Source: CAD feature listing. Evaluate the final solid. Frame: model axes, mm. Face numbers are marked on the shaded views. A direction names the side the tool comes from. Round coordinates to 2 decimals unless told otherwise and drop trailing zeros. Write each loop counter-clockwise with the first axis right and the second up, starting at its lowest first coordinate (ties: lowest second). Pieces come first, ordered by that corner, then holes.
Autodesk Inventor part; units mm, degrees
ref_plane "YZ Plane" through (0, 0, 0) normal (1, 0, 0) x (0, 1, 0)
ref_plane "XZ Plane" through (0, 0, 0) normal (0, 1, 0) x (-1, 0, 0)
ref_plane "XY Plane" through (0, 0, 0) normal (0, 0, 1) x (1, 0, 0)
sketch "Sketch1" plane through (0, 0, 0) normal (0, 1, 0) x (-1, 0, 0)
  circle A0 centre (0, 0) radius 15
  circle A1 centre (0, 0) radius 23.5
  circle A2 centre (0, 0) radius 15.5
  circle A3 centre (0, 0) radius 23
  dimension "d0" = 30
  dimension "d1" = 47
  dimension "d2" = 0.5
  dimension "d3" = 0.5
extrude "Extrusion1" add sketch "Sketch1" along normal mid plane 11 contours A1 | A2 | A3
extrude "Extrusion2" cut sketch "Sketch1" along normal mid plane 4
properties part number "Thrust Bearing 51106 - 30x47x11mm" material "Stainless Steel"
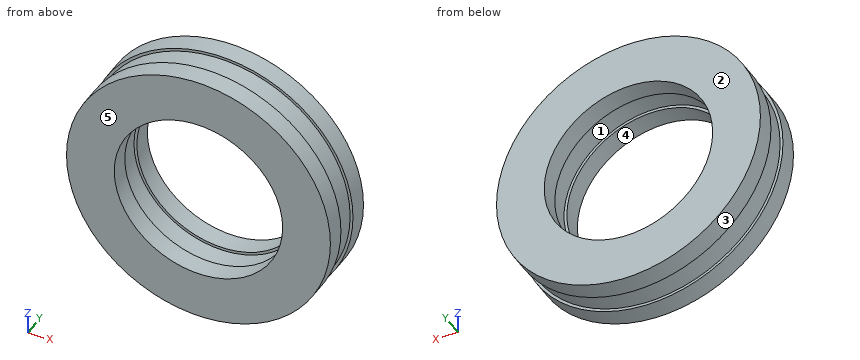
Q1. Section query D-D, the plane x = 21.5. Output: boundary loops of the cut face in (y, z).
Q2. Line query: line 1 (Z direction, x = 0, y = 4.05); line 2 (X direction, y = -4.25, z = -12.5); line 3 (Z direction, x = -5, y = -3.75). Output: solid intervals per line, ascending.
Q3. Set-up query: the marked faces 1 and 2. Return all of +Z, -Z, +X, -X, +Y, -Y with unobstructed straight access to the full face (end or side cutting, diameter ignored); none if empty.
Q4. Section query B-B, the plane x = 0. Output: boundary loops of the cut face in (y, z).
Q5. Mould query, pull axis Z, two halves, no side actions, for the marked faces 3, 4 and 5. Classes: pulls with the +Z half, pulls with the -Z half, needs draft (parallel to the pull), parting line crosses it, or undercut.
Q6. Pin query (flat end, axial travel): P1, Ø4, axis at x = -13.5, y = -2.5, coming from the -Z side; P2, Ø2, axis at x = 0.5, y = -0.5, coming from the +Z side; P3, Ø25, axis at x = -5.5, z = 4, coming from the +Y side; P4, Ø1, axis at y = 4, z = -17.5, coming from the +X side (3 decimals). Return the tip coordinate at first contact, or that it passes through.
Q7. Section query A-A, the plane z = 0. Output: boundary loops of the cut face in (x, y).
Q8. Section query C-C, the plane y = 4.25. Output: boundary loops of the cut face in (x, z), and give its area (3 significant figures).
Filled in:
1. outline: (-5.5, -9.49) - (-2, -9.49) - (-2, -8.17) - (2, -8.17) - (2, -9.49) - (5.5, -9.49) - (5.5, 9.49) - (2, 9.49) - (2, 8.17) - (-2, 8.17) - (-2, 9.49) - (-5.5, 9.49) - close
2. line 1: z = -23.5 to -15, 15 to 23.5
2. line 2: x = -19.9 to -8.29, 8.29 to 19.9
2. line 3: z = -22.96 to -14.14, 14.14 to 22.96
3. face 1: none
3. face 2: +Z, -Z, +X, -X, +Y
4. outline: (-5.5, -23.5) - (-2, -23.5) - (-2, -23) - (2, -23) - (2, -23.5) - (5.5, -23.5) - (5.5, -15) - (2, -15) - (2, -15.5) - (-2, -15.5) - (-2, -15) - (-5.5, -15) - close; (-5.5, 15) - (-2, 15) - (-2, 15.5) - (2, 15.5) - (2, 15) - (5.5, 15) - (5.5, 23.5) - (2, 23.5) - (2, 23) - (-2, 23) - (-2, 23.5) - (-5.5, 23.5) - close
5. face 3: parting line crosses it
5. face 4: undercut
5. face 5: needs draft
6. P1: stops at z = -20.49
6. P2: stops at z = 23
6. P3: stops at y = 5.5
6. P4: stops at x = 16.225
7. outline: (-23.5, -5.5) - (-15, -5.5) - (-15, -2) - (-15.5, -2) - (-15.5, 2) - (-15, 2) - (-15, 5.5) - (-23.5, 5.5) - (-23.5, 2) - (-23, 2) - (-23, -2) - (-23.5, -2) - close; (15, -5.5) - (23.5, -5.5) - (23.5, -2) - (23, -2) - (23, 2) - (23.5, 2) - (23.5, 5.5) - (15, 5.5) - (15, 2) - (15.5, 2) - (15.5, -2) - (15, -2) - close
8. outline: circle Ø47 at (0, 0); hole circle Ø30 at (0, 0)
8. area: 1,030 mm2
